```python
from build123d import *

# Parameters (mm, degrees)
BOSS_EXTRUDE1_DEPTH = 4
SKETCH2_R           = 2
SKETCH2_R_2         = 1.5
CUT_EXTRUDE1_DEPTH  = 20
SKETCH3_R           = 1.5
CUT_EXTRUDE2_DEPTH  = 10
SKETCH5_R           = 1.5
SKETCH5_R_2         = 2
CUT_EXTRUDE3_DEPTH  = 222.452026408
SKETCH7_R           = 1.5
CUT_EXTRUDE4_DEPTH  = 10


with BuildPart() as part:
    # Sketch1 → Boss-Extrude1 (new body)
    with BuildSketch(Plane.XY):
        with BuildLine():
            Line((-95, -115), (-95, -195))
            ThreePointArc((-95, -195), (-93.535533906, -198.535533906), (-90, -200))
            Line((-90, -200), (90, -200))
            ThreePointArc((90, -200), (93.535533906, -198.535533906), (95, -195))
            Line((95, -195), (95, -115))
            ThreePointArc((95, -115), (93.535533906, -111.464466094), (90, -110))
            Line((90, -110), (60, -110))
            ThreePointArc((60, -110), (56.464466094, -108.535533906), (55, -105))
            Line((55, -105), (55, -45))
            ThreePointArc((55, -45), (56.464466094, -41.464466094), (60, -40))
            Line((60, -40), (90, -40))
            ThreePointArc((90, -40), (93.535533906, -38.535533906), (95, -35))
            Line((95, -35), (95, -5))
            ThreePointArc((95, -5), (93.535533906, -1.464466094), (90, 0))
            Line((90, 0), (-90, 0))
            ThreePointArc((-90, 0), (-93.535533906, -1.464466094), (-95, -5))
            Line((-95, -5), (-95, -35))
            ThreePointArc((-95, -35), (-93.535533906, -38.535533906), (-90, -40))
            Line((-90, -40), (-60, -40))
            ThreePointArc((-60, -40), (-56.464466094, -41.464466094), (-55, -45))
            Line((-55, -45), (-55, -105))
            ThreePointArc((-55, -105), (-56.464466094, -108.535533906), (-60, -110))
            Line((-60, -110), (-90, -110))
            ThreePointArc((-90, -110), (-93.535533906, -111.464466094), (-95, -115))
        make_face()
    extrude(amount=BOSS_EXTRUDE1_DEPTH)

    # Sketch2 → Cut-Extrude1 (cut)
    with BuildSketch(Plane.XY.offset(4)):
        with Locations((-85, -185)):
            Circle(SKETCH2_R)
        with Locations((-85, -15)):
            Circle(SKETCH2_R)
        with Locations((85, -15)):
            Circle(SKETCH2_R)
        with Locations((85, -185)):
            Circle(SKETCH2_R)
        with Locations((-6.765, -180)):
            Circle(SKETCH2_R_2)
        with Locations((6.765, -180)):
            Circle(SKETCH2_R_2)
    extrude(amount=-CUT_EXTRUDE1_DEPTH, mode=Mode.SUBTRACT)

    # Sketch3 → Cut-Extrude2 (cut)
    with BuildSketch(Plane.XY.offset(4)):
        with Locations((-71.25, -75)):
            Circle(SKETCH3_R)
        with Locations((-71.25, -175)):
            Circle(SKETCH3_R)
        with Locations((-71.25, -125)):
            Circle(SKETCH3_R)
        with Locations((71.25, -75)):
            Circle(SKETCH3_R)
        with Locations((-23.75, -125)):
            Circle(SKETCH3_R)
        with Locations((-23.75, -175)):
            Circle(SKETCH3_R)
        with Locations((-47.5, -125)):
            Circle(SKETCH3_R)
        with Locations((-47.5, -175)):
            Circle(SKETCH3_R)
    extrude(amount=-CUT_EXTRUDE2_DEPTH, mode=Mode.SUBTRACT)

    # Sketch5 → Cut-Extrude3 (cut, through all)
    with BuildSketch(Plane.XY.offset(4)):
        with Locations((-40, -60)):
            Circle(SKETCH5_R)
        with Locations((-40, -80)):
            Circle(SKETCH5_R)
        with Locations(Location((40, -80, 0), (0, 0, 180))):
            Circle(SKETCH5_R)
        with Locations(Location((40, -60, 0), (0, 0, 180))):
            Circle(SKETCH5_R)
        with Locations((25.1, -132.9)):
            Circle(SKETCH5_R)
        with Locations((20, -185)):
            Circle(SKETCH5_R)
        with Locations((68.2, -183.7)):
            Circle(SKETCH5_R)
        with Locations((53, -132.9)):
            Circle(SKETCH5_R)
        with Locations((0, -7)):
            Circle(SKETCH5_R_2)
        with Locations((0, -40)):
            Circle(SKETCH5_R_2)
        with Locations((-37, -23.5)):
            Circle(SKETCH5_R)
        with Locations((37, -23.5)):
            Circle(SKETCH5_R)
    extrude(amount=-CUT_EXTRUDE3_DEPTH, mode=Mode.SUBTRACT)

    # Sketch7 → Cut-Extrude4 (cut)
    with BuildSketch(Plane(origin=(0, 0, 0), x_dir=(-1, 0, 0), z_dir=(0, 0, -1))):
        with Locations((22, -66.977361043)):
            Circle(SKETCH7_R)
        with Locations((22.009190814, -76.97735682)):
            Circle(SKETCH7_R)
        with Locations(Location((-22.009190814, -76.97735682, 0), (0, 0, 180))):
            Circle(SKETCH7_R)
        with Locations(Location((-22, -66.977361043, 0), (0, 0, 180))):
            Circle(SKETCH7_R)
        with Locations((0, -70.97735682)):
            Circle(SKETCH7_R)
        with BuildLine():
            Line((17, -120), (-17, -120))
            ThreePointArc((-17, -120), (-19.121320344, -119.121320344), (-20, -117))
            Line((-20, -117), (-20, -93))
            ThreePointArc((-20, -93), (-19.121320344, -90.878679656), (-17, -90))
            Line((-17, -90), (17, -90))
            ThreePointArc((17, -90), (19.121320344, -90.878679656), (20, -93))
            Line((20, -93), (20, -117))
            ThreePointArc((20, -117), (19.121320344, -119.121320344), (17, -120))
        make_face()
        Polygon((16, -62.977361043), (6, -62.977361043), (6, -68.977361043), (7.75, -82.977361043), (14.25, -82.977361043), (16, -68.977361043), align=None)
        Polygon((-6, -68.977361043), (-7.75, -82.977361043), (-14.25, -82.977361043), (-16, -68.977361043), (-16, -62.977361043), (-6, -62.977361043), align=None)
    extrude(amount=-CUT_EXTRUDE4_DEPTH, mode=Mode.SUBTRACT)


solid = part.part
```
Can you work these out from the model? Positions are in its coordinate system, mm. A direction names the side the tool comes from. Round coordinates to 2 decimals unless told otherwise and drop trailing zeros. Order: outer loops, then holes, each group sorted by start corner. A loop starts at its lowest first (then second) coordinate and runs counter-clockwise, first axis right, second up. Notation, with made-up numbers: (-9, 50) -> (22, 50) arc R10 ccw to (22, 62) -> close; hole circle Ø1 at (7.25, 23.25). An arc over 180 degrees is marked (long way). Return JSON: item names as keys, results as strings. Group by question number.
1. We'd pull the mould along X, two halves only. Please class faces 4 (the face through (-94, -198, 2)), 5 (the face through (93, -199, 2)), 6 (the face through (-1, -121, 0)): released by +X, released by -X, zero draft, split by the parting line, or undercut.
2. Which directions (+Z, -Z, +X, -X, +Y, -Y) give clear straight access to the entire face, cutting with the end or side of a thin tool? Please do faces 1 (the face through (56, -42, 2)), 2 (the face through (94, -2, 2)), 3 (the face through (-56, -108, 2)).
3. I need wall thicknesses on line 1 (X direction, y = -125, z = 2.1); line 2 (Y direction, x = 37, z = 1.45); line 3 (Y direction, x = -79.5, z = 3.65). Which ranges of each line are inside material? Lowest first, please. Write a range as [from, to].
4. If we section it at B-B, the plane z = 2.95: Count the separate pieces of the cut face and the enclosed holes in it, then the cut area to 3 significant figures.
5. If we section it at A-A, the plane x = -64: Write out the boundary of the cut face in (y, z).
6. Will this pin go through, and if not, where does the flat tip stop? pin 1 (2.5 mm diameter, centred on x = -40, y = -60, fed in from +Z).
Output values:
{
 "1": {"face 4": "released by -X", "face 5": "released by +X", "face 6": "zero draft"},
 "2": {"face 1": "+Z, -Z, +X", "face 2": "+Z, -Z, +X, +Y", "face 3": "+Z, -Z, -X"},
 "3": {"line 1": "[-95, -72.75], [-69.75, -49], [-46, -25.25], [-22.25, 95]", "line 2": "[-200, -25], [-22, 0]", "line 3": "[-200, -110], [-40, 0]"},
 "4": {"separate pieces": "1", "enclosed holes": "32", "area": "30,600 mm²"},
 "5": {"outline": "(-200, 0) -> (-110, 0) -> (-110, 4) -> (-200, 4) -> close; (-40, 0) -> (0, 0) -> (0, 4) -> (-40, 4) -> close"},
 "6": {"pin 1": "through"}
}
